For this review, take the finished solid that the model builds, in its own axes (mm). A direction names the side the tool comes from. Give positions to 0.01 mm unless a question says otherwise; leave off trailing zeros. Order: outer loops, then holes, each group sorted by start corner. A loop starts at its lowest first (then second) coordinate and runs counter-clockwise, first axis right, second up.
Item 1: Machinability: for faces 1 (the flat face through (-5, 36, 0.5)), 2 (the flat face through (0, -22.815, 1)), 3 (the flat face through (0, -26, -6)), which of the approach directions +Z, -Z, +X, -X, +Y, -Y give a long, thin tool a straight path to every point of the face, cutting with its end or side? Answer none if there is none.
Item 2: For P1, Ø3.5, axis at x = 5.66, y = 34.89, coming from the -Z side; P2, Ø3, axis at x = 2, z = -5, coming from the +Y side (3 decimals); P3, Ø1.2, axis at x = 6.5, y = 24.5, coming from the +Z side, all flat-tipped, find the tip position at first contact; note any pin that passes through.
Item 3: Consider section D-D (x = -8.5). Give the boundary of the cut face in (y, z) (3 decimals), plus the area to 3 significant figures.
Item 4: Consider section C-C (z = -4.25). Give the boundary of the cut face in (x, y) (3 decimals).
Item 5: Consider section B-B (x = 0). Give the boundary of the cut face in (y, z) (3 decimals), plus the area to 3 significant figures.
Item 6: Consider section A-A (y = -8.5). Give the boundary of the cut face in (x, z), plus the area to 3 significant figures.
Item 7: For probe 1 along X at (y, z) = (16.5, 2.5); probe 2 along Y at (x, z) = (-6, 2.5) (3 decimals); probe 3 along X at (y, z) = (29.5, 0.25), list the stretches that pass through material, from the lowest coordinate up.
Item 8: The part is to be moulded in two halves that separate along X. For faces 4 (the flat face through (5, 29, -0.5)), 5 (the cylindrical face through (-0.53, 33.3, 1.27)), 6 (the flat face through (-11, -7, 1)), say which applies: released by +X, released by -X, zero draft, split by the parting line, or undercut.
```python
from build123d import *

# Parameters (mm, degrees)
BOSS_EXTRUDE1_DEPTH = 3
BOSS_EXTRUDE2_START = -0.5
SKETCH1_3_R         = 11
BOSS_EXTRUDE2_DEPTH = 0.5
SKETCH2_R           = 4.1
SKETCH2_R_2         = 1.1
CUT_EXTRUDE1_DEPTH  = 3.5
SKETCH2_3_R         = 2
CUT_EXTRUDE2_DEPTH  = 2.5
CIRPATTERN2_COUNT   = 4
SKETCH1_6_W         = 11
SKETCH1_6_H         = 5.42
BOSS_EXTRUDE3_DEPTH = 6
SKETCH3_R           = 1.1
CUT_EXTRUDE3_DEPTH  = 9
SKETCH3_3_R         = 2
SKETCH3_3_R_2       = 1.1
CUT_EXTRUDE4_DEPTH  = 8


with BuildPart() as part:
    # Sketch1 → Boss-Extrude1 (new body)
    with BuildSketch(Plane.XY):
        with BuildLine():
            Line((-11, 29.235), (-11, -29.235))
            Line((-11, -29.235), (11, -29.235))
            Line((11, -29.235), (11, 29.235))
            ThreePointArc((11, 29.235), (0, 40.235), (-11, 29.235))
        make_face()
        with BuildLine():
            Line((5, -22.815), (-5, -22.815))
            Line((-5, -22.815), (-5, 18.878842411))
            ThreePointArc((-5, 18.878842411), (0, 17.735), (5, 18.878842411))
            Line((5, 18.878842411), (5, -22.815))
        make_face(mode=Mode.SUBTRACT)
    extrude(amount=BOSS_EXTRUDE1_DEPTH)

    # Sketch1<3> → Boss-Extrude2 (add)
    with BuildSketch(Plane.XY.offset(BOSS_EXTRUDE2_START)):
        with Locations((0, 29.235)):
            Circle(SKETCH1_3_R)
    extrude(amount=BOSS_EXTRUDE2_DEPTH)

    # Sketch2 → Cut-Extrude1 (cut)
    with BuildSketch(Plane.XY.offset(3)):
        with Locations((0, 29.235)):
            Circle(SKETCH2_R)
        with Locations((5.656854249, 34.891854249)):
            Circle(SKETCH2_R_2)
    cut_extrude1 = extrude(amount=-CUT_EXTRUDE1_DEPTH, mode=Mode.SUBTRACT)

    # Sketch2<3> → Cut-Extrude2 (cut)
    with BuildSketch(Plane.XY.offset(3)):
        with Locations((5.656854249, 34.891854249)):
            Circle(SKETCH2_3_R)
    cut_extrude2 = extrude(amount=-CUT_EXTRUDE2_DEPTH, mode=Mode.SUBTRACT)

    # CirPattern2: Cut-Extrude1, Cut-Extrude2 ×4 about axis
    cirpattern2_axis = Axis((0, 29.235, 0), (0, 0, 1))
    add([cut_extrude1.rotate(cirpattern2_axis, i * 360 / CIRPATTERN2_COUNT) for i in range(1, CIRPATTERN2_COUNT)], mode=Mode.SUBTRACT)
    add([cut_extrude2.rotate(cirpattern2_axis, i * 360 / CIRPATTERN2_COUNT) for i in range(1, CIRPATTERN2_COUNT)], mode=Mode.SUBTRACT)

    # Sketch1<6> → Boss-Extrude3 (add)
    with BuildSketch(Plane.XY):
        with Locations((-5.5, -26.525)):
            Rectangle(SKETCH1_6_W, SKETCH1_6_H)
        with Locations((5.5, -26.525)):
            Rectangle(SKETCH1_6_W, SKETCH1_6_H)
    extrude(amount=-BOSS_EXTRUDE3_DEPTH)

    # Sketch3 → Cut-Extrude3 (cut)
    with BuildSketch(Plane.XY.offset(3)):
        with Locations((-8.5, -26.62018786)):
            Circle(SKETCH3_R)
        with Locations((8.5, -26.62018786)):
            Circle(SKETCH3_R)
    extrude(amount=-CUT_EXTRUDE3_DEPTH, mode=Mode.SUBTRACT)

    # Sketch3<3> → Cut-Extrude4 (cut)
    # profile 1 of 2: a face of its own
    with BuildSketch(Plane.XY.offset(3)):
        with Locations((-8.5, -26.62018786)):
            Circle(SKETCH3_3_R)
        with Locations((-8.5, -26.62018786)):
            Circle(SKETCH3_3_R_2, mode=Mode.SUBTRACT)
    # profile 2 of 2: a face of its own
    with BuildSketch(Plane.XY.offset(3)):
        with Locations((8.5, -26.62018786)):
            Circle(SKETCH3_3_R)
        with Locations((8.5, -26.62018786)):
            Circle(SKETCH3_3_R_2, mode=Mode.SUBTRACT)
    extrude(amount=-CUT_EXTRUDE4_DEPTH, mode=Mode.SUBTRACT)


solid = part.part
```
Resolved:
1. face 1: +Z
1. face 2: +Z, -Z
1. face 3: -Z, +X, -X, +Y, -Y
2. P1: stops at z = -0.5
2. P2: stops at y = -23.815
2. P3: stops at z = 0.5
3. outline: (-29.235, -6) - (-27.72, -6) - (-27.72, -5) - (-28.62, -5) - (-28.62, 3) - (-29.235, 3) - close; (-25.52, -6) - (-23.815, -6) - (-23.815, 0) - (22.253, 0) - (22.253, -0.5) - (36.217, -0.5) - (36.217, 3) - (-24.62, 3) - (-24.62, -5) - (-25.52, -5) - close
3. area: 202 mm2
4. outline: (-11, -29.235) - (11, -29.235) - (11, -23.815) - (-11, -23.815) - close; hole circle Ø4 at (-8.5, -26.62); hole circle Ø4 at (8.5, -26.62)
5. outline: (-29.235, -6) - (-23.815, -6) - (-23.815, 0) - (-22.815, 0) - (-22.815, 3) - (-29.235, 3) - close; (17.735, 0) - (18.235, 0) - (18.235, -0.5) - (25.135, -0.5) - (25.135, 3) - (17.735, 3) - close; (33.335, -0.5) - (40.235, -0.5) - (40.235, 3) - (33.335, 3) - close
5. area: 102 mm2
6. outline: (-11, 0) - (-5, 0) - (-5, 3) - (-11, 3) - close; (5, 0) - (11, 0) - (11, 3) - (5, 3) - close
6. area: 36.0 mm2
7. probe 1: x = -11 to -5, 5 to 11
7. probe 2: y = -29.235 to 21.608, 25.548 to 32.922, 36.862 to 38.455
7. probe 3: x = -11 to -4.09, 4.09 to 11
8. face 4: zero draft
8. face 5: undercut
8. face 6: released by -X
